Here's the drawing with two shaded views (mm, measured from the low corner). I have some questions. Give positions to 0.01 mm unless a question says otherwise; leave off trailing zeros. Write each loop counter-clockwise with the first axis right and the second up, starting at its lowest first coordinate (ties: lowest second). Pieces come first, ordered by that corner, then holes. Notation, with made-up numbers: (71, 25.25) -> (120, 25.25) arc R20 cw to (120, 59.25) -> close; hole circle Ø7 at (-13.75, 50.5). An arc over 180 degrees is marked (long way). One line per item, written item: value.
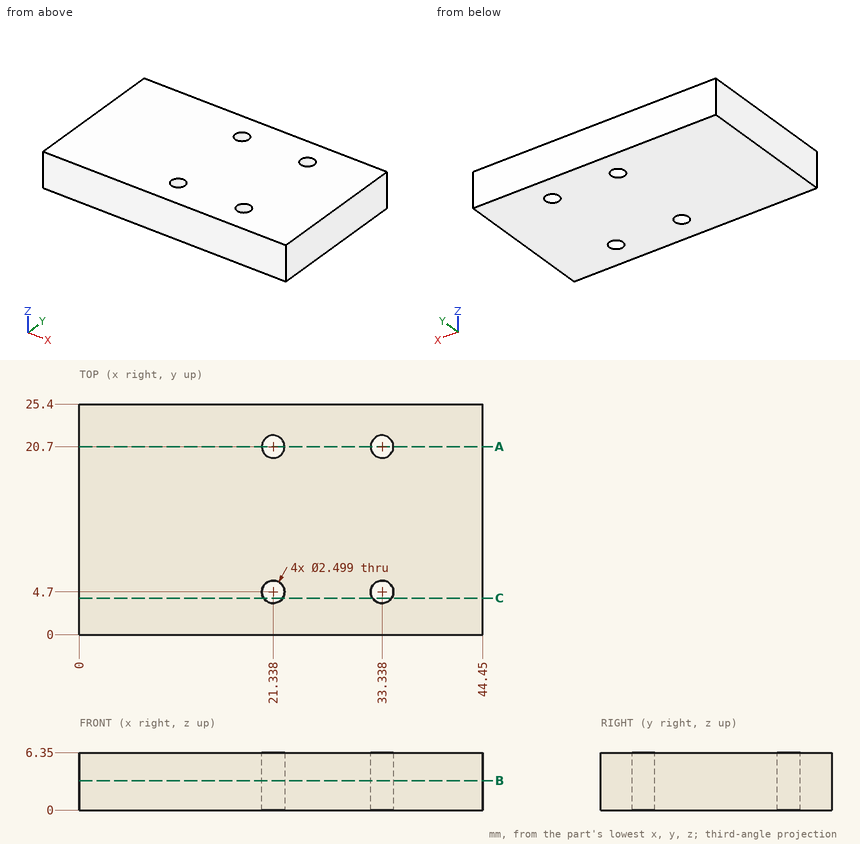
1) If we section it at A-A (y = 20.7): Write out the boundary of the cut face in (x, z).
Answer list:
outline: (0, 0) -> (20.09, 0) -> (20.09, 6.35) -> (0, 6.35) -> close; (22.59, 0) -> (32.09, 0) -> (32.09, 6.35) -> (22.59, 6.35) -> close; (34.59, 0) -> (44.45, 0) -> (44.45, 6.35) -> (34.59, 6.35) -> close
2) Will these pins go through, and if not, where does the flat tip stop? pin 1 (6 mm diameter, centred on x = 6.5, y = 13, fed in from -Z); pin 2 (2 mm diameter, centred on x = 21.34, y = 20.7, fed in from -Z).
Answer list:
pin 1: stops at z = 0
pin 2: passes through
3) I need wall thicknesses on L1, parallel to X at y = 4.7, z = 5; L2, parallel to Y at x = 21, z = 3.25; L3, parallel to Y at x = 34, z = 3.25. Which ranges of each line are inside material? Lowest first, please.
Answer list:
L1: x = 0 to 20.09, 22.59 to 32.09, 34.59 to 44.45
L2: y = 0 to 3.5, 5.9 to 19.5, 21.9 to 25.4
L3: y = 0 to 3.64, 5.76 to 19.64, 21.76 to 25.4
4) If we section it at C-C (y = 4): Write out the boundary of the cut face in (x, z).
Answer list:
outline: (0, 0) -> (20.3, 0) -> (20.3, 6.35) -> (0, 6.35) -> close; (22.37, 0) -> (32.3, 0) -> (32.3, 6.35) -> (22.37, 6.35) -> close; (34.37, 0) -> (44.45, 0) -> (44.45, 6.35) -> (34.37, 6.35) -> close
5) If we section it at B-B (z = 3.25): Write out the boundary of the cut face in (x, y).
Answer list:
outline: (0, 0) -> (44.45, 0) -> (44.45, 25.4) -> (0, 25.4) -> close; hole circle Ø2.5 at (21.34, 4.7); hole circle Ø2.5 at (21.34, 20.7); hole circle Ø2.5 at (33.34, 4.7); hole circle Ø2.5 at (33.34, 20.7)
